Here's how the part is built. I have some questions about the finished solid (model axes, mm). Round coordinates to 2 decimals unless told otherwise and drop trailing zeros. Order: outer loops, then holes, each group sorted by start corner. A loop starts at its lowest first (then second) coordinate and runs counter-clockwise, first axis right, second up. Notation, with made-up numbers: (74.25, 64.5) - (99.25, 64.5) arc R23 ccw to (99.25, 77.5) - close; hole circle Ø8 at (9.25, -17). An arc over 180 degrees is marked (long way). Answer as a JSON object with one key per item and string values.
```python
from build123d import *

# Parameters (mm, degrees)
F0_R     = 0.4318
F0_R_2   = 0.3556
F1_DEPTH = 508
F3_R     = 0.762
F4_DEPTH = 6.096


with BuildPart() as f1:
    # F0 (on Front) → F1 (new body)
    with BuildSketch(Plane.XZ):
        Circle(F0_R)
        Circle(F0_R_2, mode=Mode.SUBTRACT)
    extrude(amount=F1_DEPTH)

    # F3 (on offset) → F4 (join)
    with BuildSketch(Plane.XZ.offset(26.3398)):
        Circle(F3_R)
    extrude(amount=F4_DEPTH)


solid = f1.part
```
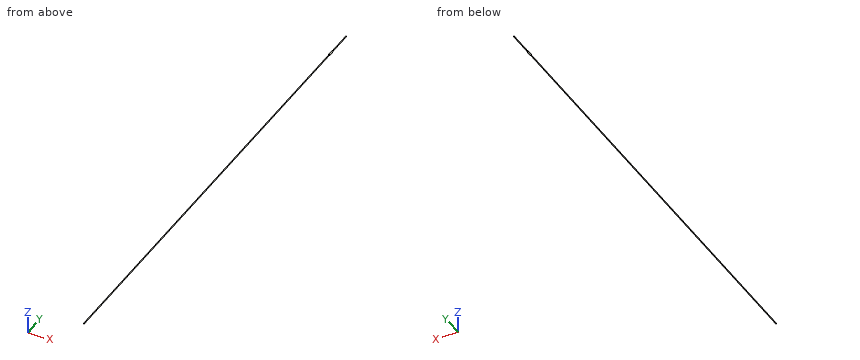
1. Imagine slicing it at B-B (x = 0). List the corners of the cut face in (y, z) for me, plus the area to 3 significant figures.
Responses:
{"outline": "(-508, -0.43) - (-32.44, -0.43) - (-32.44, -0.76) - (-26.34, -0.76) - (-26.34, -0.43) - (0, -0.43) - (0, -0.36) - (-26.34, -0.36) - (-26.34, 0.36) - (0, 0.36) - (0, 0.43) - (-26.34, 0.43) - (-26.34, 0.76) - (-32.44, 0.76) - (-32.44, 0.43) - (-508, 0.43) - (-508, 0.36) - (-32.44, 0.36) - (-32.44, -0.36) - (-508, -0.36) - close", "area": "85.8 mm2"}
2. If I drill on L1, parallel to Y at x = 0.2, z = 0.45, over which ranges is the centre line in solid material (lowest first)? Write a range as [from, to].
Responses:
{"L1": "[-32.44, -26.34]"}
3. Imagine slicing it at A-A (z = 0). List the corners of the cut face in (x, y) for me, plus the area to 3 significant figures.
Responses:
{"outline": "(-0.76, -32.44) - (-0.43, -32.44) - (-0.43, -508) - (-0.36, -508) - (-0.36, -32.44) - (0.36, -32.44) - (0.36, -508) - (0.43, -508) - (0.43, -32.44) - (0.76, -32.44) - (0.76, -26.34) - (0.43, -26.34) - (0.43, 0) - (0.36, 0) - (0.36, -26.34) - (-0.36, -26.34) - (-0.36, 0) - (-0.43, 0) - (-0.43, -26.34) - (-0.76, -26.34) - close", "area": "85.8 mm2"}
